Here's how the part is built. I have some questions about the finished solid (model axes, mm). Face numbers are marked on the shaded views. A direction names the side the tool comes from. Give positions to 0.01 mm unless a question says otherwise; leave off trailing zeros. Loops run counter-clockwise (first coordinate to the right, second up) from the corner with the lowest first, then second, coordinate; pieces in that order, holes last. Notation, with made-up numbers: (14.25, -16) - (39.25, -16) arc R30 ccw to (39.25, 20) - close; hole circle Ø5 at (41, -14.5). An arc over 180 degrees is marked (long way). Put each result on its own line as item: value. Start each with the question number.
from build123d import *

# Parameters (mm, degrees)
F0_W     = 50
F0_H     = 20
F0_R     = 3
F1_DEPTH = 10
F2_W     = 42
F2_H     = 55
F3_DEPTH = 20
F4_W     = 3
F4_H     = 20
F4_H_2   = 45
F5_DEPTH = 20
F6_W     = 15
F6_H     = 25
F7_DEPTH = 10


# Not quite as in the source:
# - a pattern or mirror of a feature is missing from the dataset's text; its kind, count and spacing are read off the source's solid


with BuildPart() as f1:
    # F0 (on Top) → F1 (new body)
    with BuildSketch(Plane.XY):
        with Locations((0, -2.5)):
            Rectangle(F0_W, F0_H)
        with Locations((-17.5, -5)):
            Circle(F0_R, mode=Mode.SUBTRACT)
        with Locations((17.5, -5)):
            Circle(F0_R, mode=Mode.SUBTRACT)
    extrude(amount=F1_DEPTH)

    # F2 (on face) → F3 (join)
    with BuildSketch(Plane(origin=(0, 7.5, 0), x_dir=(-1, 0, 0), z_dir=(0, 1, 0))):
        with Locations((0, 37.5)):
            Rectangle(F2_W, F2_H)
    extrude(amount=-F3_DEPTH)

    # F4 (on face) → F5 (cut, through all)
    with BuildSketch(Plane(origin=(0, 7.5, 0), x_dir=(-1, 0, 0), z_dir=(0, 1, 0))):
        with Locations((-15, 50)):
            Rectangle(F4_W, F4_H)
        with Locations((0, 37.5)):
            Rectangle(F4_W, F4_H_2)
        with Locations((15, 50)):
            Rectangle(F4_W, F4_H)
    extrude(amount=-F5_DEPTH, mode=Mode.SUBTRACT)

    # F6 (on face) → F7 (cut)
    with BuildSketch(Plane.YZ.offset(21)):
        with Locations((-5, 22.5)):
            Rectangle(F6_W, F6_H)
    f7 = extrude(amount=-F7_DEPTH, mode=Mode.SUBTRACT)

    # F7_copies: F7 across plane
    add(f7.mirror(Plane(origin=(0, 0, 0), x_dir=(0, 0, -1), z_dir=(-1, 0, 0))), mode=Mode.SUBTRACT)


solid = f1.part
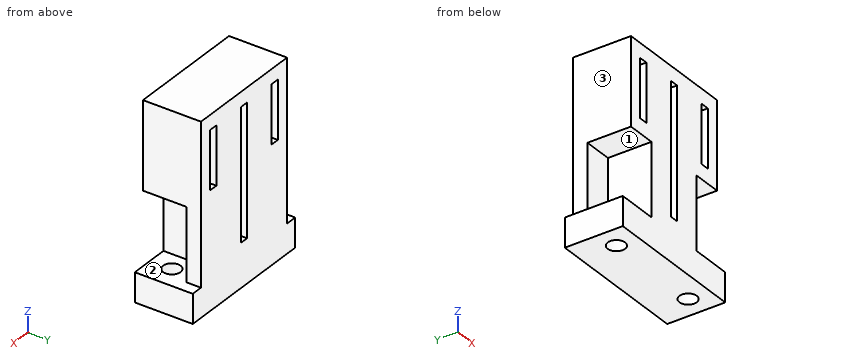
1) I need wall thicknesses on line 1 (X direction, y = 4.5, z = 52.5); line 2 (Z direction, x = -14.5, y = -11); line 3 (Z direction, x = -1, y = -2.5). Which ranges of each line are inside material? Lowest first, please.
2) Suppose I cut it at A-A on y = -5. Give the number of separate pieces and of enclosed holes in the cut face, plus the area to 4 significant figures.
3) Suppose I cut it at C-C on z = 16. Please give me the cut outline in (x, y).
4) Suppose I cut it at D-D on y = 0. Please give me the cut outline in (x, z), plus the area to 4 significant figures.
5) Which directions (+Z, -Z, +X, -X, +Y, -Y) give clear straight access to the entire face, cutting with the end or side of a thin tool? Please do the marked faces 1, 2 and 3.
6) I'm going to push flat-ended pins straight in: P1, Ø1.5, axis at x = -1, y = -3.5, coming from the -Z side; P2, Ø7.5, axis at y = -6.5, z = 22.5, coming from the -X side; P3, Ø5, axis at x = -14.5, z = 22.5, coming from the -Y side; P4, Ø10, axis at y = 0, z = 37, coming from the -X side. Where does each tip first touch, or does it pass through?
7) Suppose I cut it at B-B on x = 17.5. Please give me the cut outline in (y, z), plus the area to 3 significant figures.
Ans:
1. line 1: x = -21 to -16.5, -13.5 to -1.5, 1.5 to 13.5, 16.5 to 21
1. line 2: z = 0 to 10, 35 to 40, 60 to 65
1. line 3: z = 0 to 15, 60 to 65
2. separate pieces: 3
2. enclosed holes: 3
2. area: 1,935 mm²
3. outline: (-21, 2.5) - (-11, 2.5) - (-11, -12.5) - (-1.5, -12.5) - (-1.5, 7.5) - (-21, 7.5) - close; (1.5, -12.5) - (11, -12.5) - (11, 2.5) - (21, 2.5) - (21, 7.5) - (1.5, 7.5) - close
4. outline: (-25, 0) - (25, 0) - (25, 10) - (11, 10) - (11, 35) - (21, 35) - (21, 65) - (-21, 65) - (-21, 35) - (-11, 35) - (-11, 10) - (-25, 10) - close; hole (-16.5, 40) - (-13.5, 40) - (-13.5, 60) - (-16.5, 60) - close; hole (-1.5, 15) - (1.5, 15) - (1.5, 60) - (-1.5, 60) - close; hole (13.5, 40) - (16.5, 40) - (16.5, 60) - (13.5, 60) - close
4. area: 2,055 mm²
5. face 1: -X, -Y
5. face 2: +X, -Y
5. face 3: +Z, -X, +Y, -Y
6. P1: stops at z = 0
6. P2: stops at x = -11
6. P3: stops at y = 2.5
6. P4: stops at x = -21
7. outline: (-12.5, 0) - (-8, 0) - (-8, 10) - (-12.5, 10) - close; (-12.5, 35) - (2.5, 35) - (2.5, 10) - (-2, 10) - (-2, 0) - (7.5, 0) - (7.5, 65) - (-12.5, 65) - close
7. area: 865 mm²
